Can you work these out from the drawing? Everything is in mm from the part's minimum corner. Coordinates: 2 decimals unless noted, no trailing zeros. Loops run counter-clockwise (first coordinate to the right, second up) from the corner with the lowest first, then second, coordinate; pieces in that order, holes last. Notation, with made-up numbers: (-7.5, -18.75) - (48.5, -18.75) arc R9 ccw to (48.5, -1.75) - close; hole circle Ø4 at (23.25, -21). An arc over 180 degrees is marked (long way). One line per question, with ' | ' between items. Start each with the question number.
1. I want a section at B-B, the plane x = 15.5. Write out the boundary of the cut face in (y, z), then the cut area to 3 significant figures.
2. I'm going to push flat-ended pins straight in: P1, Ø3, axis at y = 14, z = 26.5, coming from the +X side; P2, Ø2.5, axis at y = 3.81, z = 22.03, coming from the +X side; P3, Ø1, axis at x = 4.5, y = 28, coming from the -Z side; P4, Ø6, axis at y = 18, z = 33.5, coming from the -X side (1 decimal). Where does each tip first touch, or does it pass through?
3. I want a section at A-A, the plane y = 3.81. Count the separate pieces of the cut face and the enclosed holes in it.
4. I want a section at C-C, the plane z = 4. Write out the boundary of the cut face in (x, y) (1 decimal).
5. We'd pull the mould along X, two halves only. Please class the marked faces 1, 2 and 3: pulls with the +X half, pulls with the -X half, needs draft (parallel to the pull), parting line crosses it, or undercut.
6. Please list where these lines run through material, in increasing order: L1, parallel to Z at x = 22, y = 11 (1 decimal); L2, parallel to X at y = 20, z = 22.5; L3, parallel to Z at x = 19, y = 28. Write a range as [from, to].
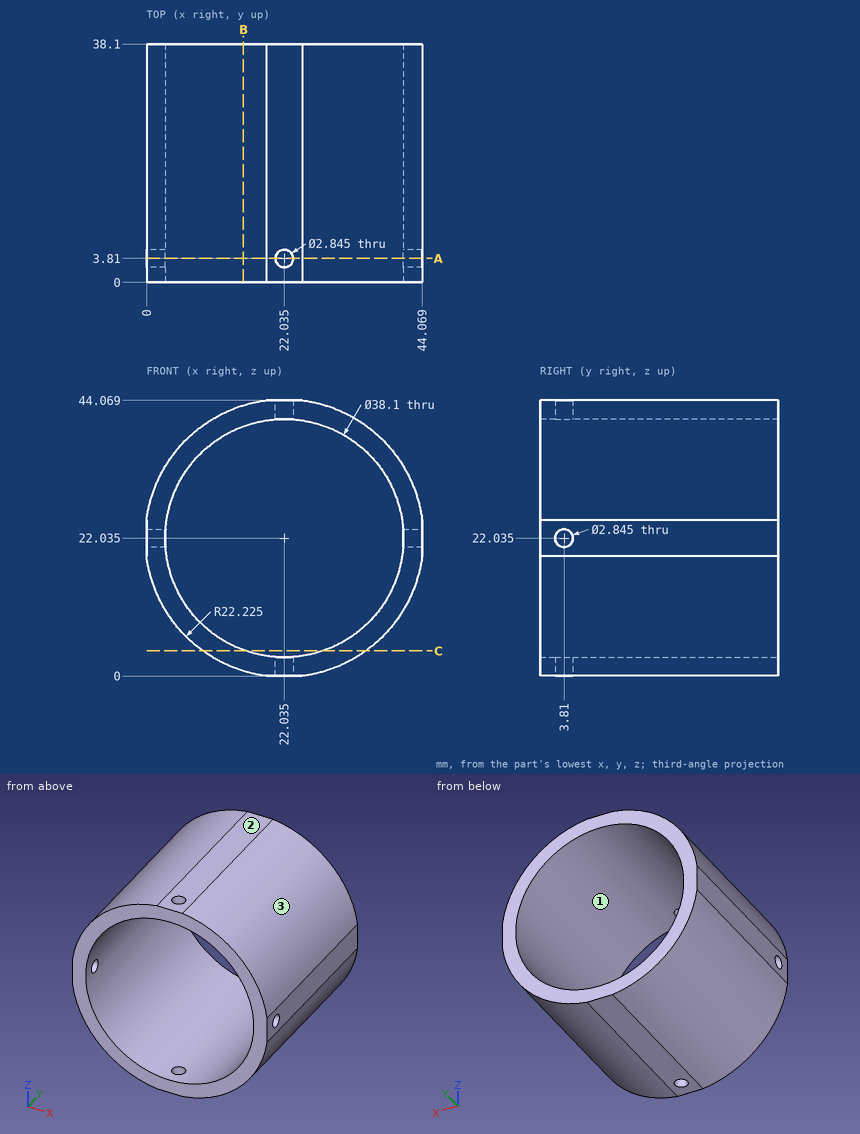
Results are:
1) outline: (0, 0.79) - (38.1, 0.79) - (38.1, 4.14) - (0, 4.14) - close; (0, 39.93) - (38.1, 39.93) - (38.1, 43.28) - (0, 43.28) - close | area: 255 mm2
2) P1: stops at x = 44.06 | P2: passes through | P3: stops at z = 7.76 | P4: stops at x = 1.5
3) separate pieces: 4 | enclosed holes: 0
4) outline: (9, 0) - (15.9, 0) - (15.9, 38.1) - (9, 38.1) - close; (28.2, 0) - (35, 0) - (35, 38.1) - (28.2, 38.1) - close
5) face 1: undercut | face 2: needs draft | face 3: pulls with the +X half
6) L1: z = [0, 3], [41.1, 44.1] | L2: x = [0, 2.99], [41.08, 44.07] | L3: z = [0.02, 3.23], [40.84, 44.05]
